Verification items for the finished model (mm, model axes). Face numbers are marked on the shaded views. A direction names the side the tool comes from. Round coordinates to 2 decimals unless told otherwise and drop trailing zeros. Write each loop counter-clockwise with the first axis right and the second up, starting at its lowest first coordinate (ties: lowest second). Pieces come first, ordered by that corner, then holes. Notation, with made-up numbers: M 57.5,-35 L 103.5,-35 A21 ccw 103.5,-30 Z; hole C 61.25,-15.5 d8. An arc over 180 degrees is marked long. Write each question's results on one line, items separated by ' | '.
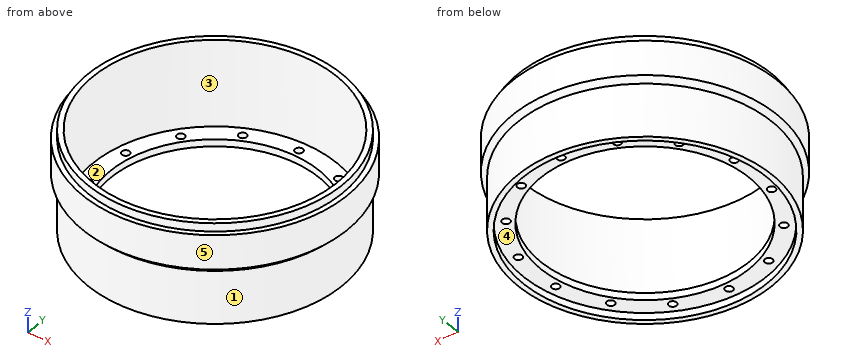
from build123d import *

# Parameters (mm, degrees)
ESQUISSE2_R             = 1.1
ENL_V_MAT_EXTRU_1_DEPTH = 59.29039372


with BuildPart() as part:
    # Esquisse1 → Révolution1 (revolve)
    with BuildSketch(Plane(origin=(0, 0, 0), x_dir=(0, 0, -1), z_dir=(1, 0, 0)), mode=Mode.PRIVATE) as r_volution1_sk:
        Polygon((0, 34.5), (0, 36), (-15, 36), (-16.4, 37.4), (-26.15, 37.4), (-26.15, 36), (-28.5, 36), (-28.5, 34.5), (-4, 34.5), (-4, 29.55), (-2, 29.55), (-2, 34.5), align=None)
    revolve(r_volution1_sk.sketch.rotate(Axis((0, 0, 14.835870703), (0, 0, -1)), 90), axis=Axis((0, 0, 14.835870703), (0, 0, -1)))

    # Esquisse2 → Enlèv. mat.-Extru.1 (cut, through all)
    with BuildSketch(Plane.XY.offset(4)):
        with Locations((0, 31.67)):
            Circle(ESQUISSE2_R)
        with Locations((13.741098018, 28.533684046)):
            Circle(ESQUISSE2_R)
        with Locations((24.76060305, 19.745922025)):
            Circle(ESQUISSE2_R)
        with Locations((30.875966979, 7.047237978)):
            Circle(ESQUISSE2_R)
        with Locations((30.875966979, -7.047237978)):
            Circle(ESQUISSE2_R)
        with Locations((24.76060305, -19.745922025)):
            Circle(ESQUISSE2_R)
        with Locations((13.741098018, -28.533684046)):
            Circle(ESQUISSE2_R)
        with Locations((0, -31.67)):
            Circle(ESQUISSE2_R)
        with Locations((-13.741098018, -28.533684046)):
            Circle(ESQUISSE2_R)
        with Locations((-24.76060305, -19.745922025)):
            Circle(ESQUISSE2_R)
        with Locations((-30.875966979, -7.047237978)):
            Circle(ESQUISSE2_R)
        with Locations((-30.875966979, 7.047237978)):
            Circle(ESQUISSE2_R)
        with Locations((-24.76060305, 19.745922025)):
            Circle(ESQUISSE2_R)
        with Locations((-13.741098018, 28.533684046)):
            Circle(ESQUISSE2_R)
    extrude(amount=-ENL_V_MAT_EXTRU_1_DEPTH, mode=Mode.SUBTRACT)


solid = part.part
1) Sectioned sample at A-A, the plane x = 0. Count the separate pieces of the cut face and the enclosed holes in it, and give its area (3 significant figures).
Calculated:
separate pieces: 4 | enclosed holes: 0 | area: 126 mm²
2) Draft check along Y on the marked faces 1 and 2. Enter one of: pulls with the +Y half, pulls with the -Y half, needs draft (parallel to the pull), parting line crosses it, or undercut.
Calculated:
face 1: parting line crosses it | face 2: undercut
3) Access from +Z, -Z, +X, -X, +Y, -Y to the whole of each face (thin tool, end or side, straight path). Record for the marked faces 3, 4 and 5.
Calculated:
face 3: +Z | face 4: -Z | face 5: +Z, -Z
4) Material ranges on line 1 (X direction, y = 10.5, z = 16.5); line 2 (Y direction, x = 30, z = 24.5); line 3 (Y direction, x = 12.5, z = 3), recorded low to high. Write a range as [from, to].
Calculated:
line 1: x = [-35.9, -32.86], [32.86, 35.9] | line 2: y = [-22.33, -17.04], [17.04, 22.33] | line 3: y = [-33.76, -26.78], [26.78, 33.76]
5) Depth check by flat-ended pin: P1, Ø1, axis at x = 26.5, z = 5.5, coming from the -Y side; P2, Ø1, axis at x = 6.5, z = 10, coming from the +Y side; P3, Ø2.5, axis at x = 30.88, y = 7.05, coming from the -Z side; P4, Ø1.8, axis at x = -24.76, y = 19.75, coming from the -Z side. Enter the tip coordinate at first touch or a pass-through.
Calculated:
P1: stops at y = -24.9 | P2: stops at y = 35.5 | P3: stops at z = 2 | P4: passes through
6) Sectioned sample at C-C, the plane z = 13. Record the cut outline in (x, y), and give its area (3 significant figures).
Calculated:
outline: C 0,0 d72; hole C 0,0 d69 | area: 332 mm²
7) Sectioned sample at B-B, the plane y = 0. Record the cut outline in (x, z), and give its area (3 significant figures).
Calculated:
outline: M -37.4,16.4 L -36,15 L -36,0 L -34.5,0 L -34.5,2 L -29.55,2 L -29.55,4 L -34.5,4 L -34.5,28.5 L -36,28.5 L -36,26.15 L -37.4,26.15 Z; M 29.55,2 L 34.5,2 L 34.5,0 L 36,0 L 36,15 L 37.4,16.4 L 37.4,26.15 L 36,26.15 L 36,28.5 L 34.5,28.5 L 34.5,4 L 29.55,4 Z | area: 135 mm²
